The drawing under review shows one solid part. Ordinate dimensions are in mm from its lowest x, y, z. Give positions to 0.01 mm unless a question says otherwise; leave off trailing zeros. Order: outer loops, then holes, each group sorted by start corner. A loop starts at its lowest first (then second) coordinate and runs counter-clockwise, first axis right, second up. Notation, with made-up numbers: (40, 54) - (74, 54) arc R12 cw to (74, 58) - close; hole circle Ø7 at (20.5, -25.75). An arc over 180 degrees is marked (long way). Write item = value, one per line. Start each with the question number.
1. For P1, Ø4.5, axis at y = 102.5, z = 9, coming from the -X side; P2, Ø10, axis at y = 111, z = 21.5, coming from the +X side, all flat-tipped, find the tip position at first contact; note any pin that passes through.
2. We need section A-A, the plane y = 76.5. Give the boundary of the cut face in (x, z).
3. Wall thickness on probe 1 along Y at (x, z) = (22.5, 15.5); probe 2 along X at (y, z) = (114, 8.25); probe 3 along Z at (x, y) = (54, 112.5): over which ranges is each line inside the solid? List them lowest first.
4. We need section B-B, the plane z = 14.75. Give the boundary of the cut face in (x, y).
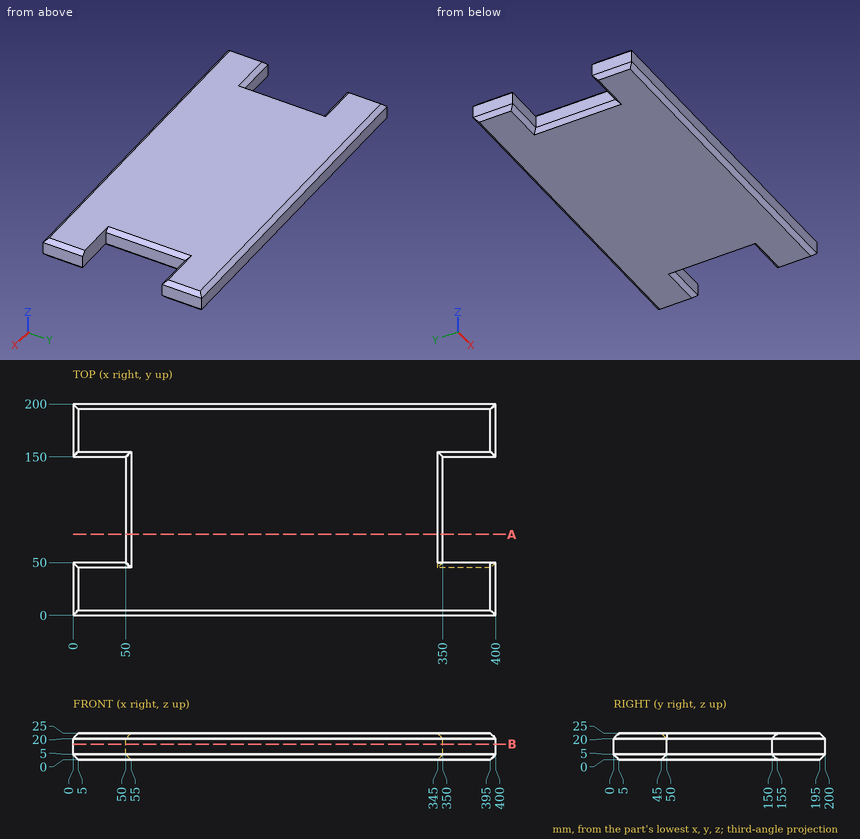
Model answer:
q1.P1 = 50
q1.P2 = 350
q2.outline = (50, 5) - (55, 0) - (345, 0) - (350, 5) - (350, 20) - (345, 25) - (55, 25) - (50, 20) - close
q3.probe_1 = 0 to 50, 150 to 200
q3.probe_2 = 50 to 350
q3.probe_3 = 1 to 24
q4.outline = (0, 0) - (400, 0) - (400, 50) - (350, 50) - (350, 150) - (400, 150) - (400, 200) - (0, 200) - (0, 150) - (50, 150) - (50, 50) - (0, 50) - close
